```python
from build123d import *

# Parameters (mm, degrees)
SKETCH1_R               = 32.5
SKETCH1_R_2             = 30
BOSS_EXTRUDE1_DEPTH     = 140
CUT_REVOLVE1_ANGLE      = 67
CUT_REVOLVE2_ANGLE      = 67
CUT_EXTRUDE1_DEPTH      = 58
CUT_EXTRUDE1_DEPTH_BACK = 50
BOSS_EXTRUDE3_START     = -70
SKETCH4_R               = 1.55
BOSS_EXTRUDE3_DEPTH     = 4
SKETCH6_W               = 19.62
SKETCH6_H               = 2.5
BOSS_EXTRUDE4_DEPTH     = 6
SKETCH7_W               = 6
SKETCH7_H               = 9.773229536
BOSS_EXTRUDE6_DEPTH     = 3
SKETCH8_W               = 2.5
SKETCH8_H               = 1.33
BOSS_EXTRUDE7_DEPTH     = 6
SKETCH9_R               = 1.1
CUT_EXTRUDE2_DEPTH      = 7
RIB3_REACH              = 156.088
SKETCH11_WALL_W         = 347.41014935
SKETCH11_WALL_H         = 6


with BuildPart() as part:
    # Sketch1 → Boss-Extrude1 (new body)
    with BuildSketch(Plane(origin=(0, 0, 0), x_dir=(1, 0, 0), z_dir=(0, 1, 0))):
        with Locations(Location((0, 0, 0), (0, 0, 270))):
            Circle(SKETCH1_R)
        with Locations(Location((0, 0, 0), (0, 0, 270))):
            Circle(SKETCH1_R_2, mode=Mode.SUBTRACT)
    extrude(amount=BOSS_EXTRUDE1_DEPTH)

    # Sketch2 → Cut-Revolve1 (revolve, cut)
    with BuildSketch(Plane.XY):
        with BuildLine():
            Line((-42.5, 107.716148379), (42.5, 107.716148379))
            ThreePointArc((42.5, 107.716148379), (0, 150.216148379), (-42.5, 107.716148379))
        make_face()
    revolve(axis=Axis((-42.5, 107.716148379, 0), (1, 0, 0)), revolution_arc=CUT_REVOLVE1_ANGLE, mode=Mode.SUBTRACT)

    # Sketch3 → Cut-Revolve2 (revolve, cut)
    with BuildSketch(Plane.XY):
        with BuildLine():
            Line((-42.5, 70.076349177), (42.5, 70.076349177))
            ThreePointArc((42.5, 70.076349177), (0, 27.576349177), (-42.5, 70.076349177))
        make_face()
    revolve(axis=Axis((-42.5, 70.076349177, 0), (1, 0, 0)), revolution_arc=CUT_REVOLVE2_ANGLE, mode=Mode.SUBTRACT)

    # Sketch5 → Cut-Extrude1 (cut, two sides)
    with BuildSketch(Plane(origin=(0, 0, 0), x_dir=(0, 0, -1), z_dir=(1, 0, 0))) as cut_extrude1_sk:
        with BuildLine():
            Line((-38.488633311, 38.604979811), (-38.087882821, 37.828391715))
            ThreePointArc((-38.087882821, 37.828391715), (-30.720780367, 29.920302027), (-20.314824517, 27))
            Line((-20.314824517, 27), (-19.990167054, 27))
            Line((-19.990167054, 27), (0, 27))
            Line((0, 27), (0, 5))
            Line((0, 5), (-38.488633311, 5))
            Line((-38.488633311, 5), (-38.488633311, 38.604979811))
        make_face()
    extrude(amount=CUT_EXTRUDE1_DEPTH, mode=Mode.SUBTRACT)
    extrude(cut_extrude1_sk.sketch, amount=-CUT_EXTRUDE1_DEPTH_BACK, mode=Mode.SUBTRACT)

    # Sketch4 → Boss-Extrude3 (add)
    with BuildSketch(Plane(origin=(0, 140, 0), x_dir=(1, 0, 0), z_dir=(0, 1, 0)).offset(BOSS_EXTRUDE3_START)):
        with BuildLine():
            Line((-2.218998773, 40.206666667), (-20.604988608, 25.133333333))
            ThreePointArc((-20.604988608, 25.133333333), (0, 32.5), (20.604988608, 25.133333333))
            Line((20.604988608, 25.133333333), (2.218998773, 40.206666667))
            ThreePointArc((2.218998773, 40.206666667), (0, 41), (-2.218998773, 40.206666667))
        make_face()
        with Locations(Location((0, 37.5, 0), (0, 0, 270))):
            Circle(SKETCH4_R, mode=Mode.SUBTRACT)
        with BuildLine():
            ThreePointArc((-25.133333333, -20.604988608), (-32.5, 0), (-25.133333333, 20.604988608))
            Line((-25.133333333, 20.604988608), (-40.206666667, 2.218998773))
            ThreePointArc((-40.206666667, 2.218998773), (-41, 0), (-40.206666667, -2.218998773))
            Line((-40.206666667, -2.218998773), (-25.133333333, -20.604988608))
        make_face()
        with Locations(Location((-37.5, 0, 0), (0, 0, 270))):
            Circle(SKETCH4_R, mode=Mode.SUBTRACT)
        with BuildLine():
            Line((40.206666667, 2.218998773), (25.133333333, 20.604988608))
            ThreePointArc((25.133333333, 20.604988608), (32.5, 0), (25.133333333, -20.604988608))
            Line((25.133333333, -20.604988608), (40.206666667, -2.218998773))
            ThreePointArc((40.206666667, -2.218998773), (41, 0), (40.206666667, 2.218998773))
        make_face()
        with Locations(Location((37.5, 0, 0), (0, 0, 270))):
            Circle(SKETCH4_R, mode=Mode.SUBTRACT)
        with BuildLine():
            ThreePointArc((20.604988608, -25.133333333), (0, -32.5), (-20.604988608, -25.133333333))
            Line((-20.604988608, -25.133333333), (-2.218998773, -40.206666667))
            ThreePointArc((-2.218998773, -40.206666667), (0, -41), (2.218998773, -40.206666667))
            Line((2.218998773, -40.206666667), (20.604988608, -25.133333333))
        make_face()
        with Locations(Location((0, -37.5, 0), (0, 0, 270))):
            Circle(SKETCH4_R, mode=Mode.SUBTRACT)
    extrude(amount=-BOSS_EXTRUDE3_DEPTH)

    # Sketch6 → Boss-Extrude4 (add)
    with BuildSketch(Plane.XY):
        with Locations((39.81, 24.42)):
            Rectangle(SKETCH6_W, SKETCH6_H)
    extrude(amount=BOSS_EXTRUDE4_DEPTH)

    # Sketch7 → Boss-Extrude6 (add)
    with BuildSketch(Plane(origin=(49.62, 0, 0), x_dir=(0, 0, -1), z_dir=(1, 0, 0))):
        with Locations((-3, 18.283385232)):
            Rectangle(SKETCH7_W, SKETCH7_H)
    extrude(amount=-BOSS_EXTRUDE6_DEPTH)

    # Sketch8 → Boss-Extrude7 (add)
    with BuildSketch(Plane.XY):
        Polygon((49.62, 25.67), (32.5, 25.67), (32.5, 27), align=None)
        with Locations((31.25, 26.335)):
            Rectangle(SKETCH8_W, SKETCH8_H)
    extrude(amount=BOSS_EXTRUDE7_DEPTH)

    # Sketch9 → Cut-Extrude2 (cut)
    with BuildSketch(Plane(origin=(49.62, 0, 0), x_dir=(0, 0, -1), z_dir=(1, 0, 0))):
        with Locations((-3, 14.913761398)):
            Circle(SKETCH9_R)
    extrude(amount=-CUT_EXTRUDE2_DEPTH, mode=Mode.SUBTRACT)

    # Sketch11 wall → Rib3 (add, up to next)
    with BuildSketch(Plane(origin=(41.06, 42.202329556, 0), x_dir=(0.459795586238, -0.888024785057, 0), z_dir=(0.888024785057, 0.459795586238, 0)), mode=Mode.PRIVATE) as rib3_sk1:
        with Locations((0, -3)):
            Rectangle(SKETCH11_WALL_W, SKETCH11_WALL_H)
    rib3_tool1 = extrude(rib3_sk1.sketch, amount=-RIB3_REACH, mode=Mode.PRIVATE) - part.part
    add(rib3_tool1.solids().sort_by_distance((41.06, 42.202329556, 0))[0])


solid = part.part
```
Geometry check sheet. Reference: the model listing, model coordinates, mm. A direction names the side the tool comes from. Round coordinates to 2 decimals unless told otherwise and drop trailing zeros. Loops run counter-clockwise (first coordinate to the right, second up) from the corner with the lowest first, then second, coordinate; pieces in that order, holes last. Notation, with made-up numbers: (-12, 73) -> (1, 73) arc R18 cw to (1, 89) -> close; hole circle Ø5 at (46, 24). An arc over 180 degrees is marked (long way). Use a Markdown table: item, result.
(1) Set-up check for faces 4 (the flat face through (46.62, 18, 3)), 5 (the flat face through (0, 5, 31)), 6 (the cylindrical face through (21.97, 69.02, -23.95)), 7 (the cylindrical face through (41, 68, 0)), 8 (the cylindrical face through (35.987, 68.028, -0.336)): record each of +Z, -Z, +X, -X, +Y, -Y from which the full face is reachable in a straight line by a thin tool's end or side.
Calculated:
| item | result |
|---|---|
| face 4 | +Z, -Z, -X, -Y |
| face 5 | +Z, +X, -X |
| face 6 | none |
| face 7 | +X, +Y |
| face 8 | +Y |
(2) Go/stop test with flat-tipped pins: P1, Ø8, axis at x = -34, z = -7, coming from the -Y side; P2, Ø2.5, axis at x = 37.5, z = 0, coming from the -Y side; P3, Ø8, axis at x = -15, y = 78.5, coming from the +Z side; P4, Ø1.9, axis at y = 25, z = 2, coming from the -X side. Record where each tip stops, or that it passes through.
Calculated:
| item | result |
|---|---|
| P1 | y = 0 |
| P2 | y = 23.17 |
| P3 | z = 30.58 |
| P4 | x = 30 |
(3) Scan lines: probe 1 along X at (y, z) = (48.5, 17); probe 2 along X at (y, z) = (74.5, 26); probe 3 along Z at (x, y) = (-37, 68). Record each from-to range of solid material in increasing order.
Calculated:
| item | result |
|---|---|
| probe 1 | -27.7 to -24.72, 24.72 to 27.7 |
| probe 2 | -19.5 to -14.97, 14.97 to 19.5 |
| probe 3 | -6.13 to -1.47, 1.47 to 6.13 |
(4) Sectioned sample at A-A (x = 12.5). Enter the section's corners in (y, z), then the cut area to 3 significant figures.
Calculated:
| item | result |
|---|---|
| outline | (0, -30) -> (42.69, -30) arc R40.62 cw to (39.97, -27.27) -> (0, -27.27) -> close; (0, 27.27) -> (5, 27.27) -> (5, 30) -> (0, 30) -> close; (28.25, 27.27) -> (119.29, 27.27) -> (120.45, 30) -> (70, 30) -> (70, 31.78) -> (66, 31.78) -> (66, 30) -> (29.5, 30) arc R20 ccw to start; (57.34, -30) -> (66, -30) -> (66, -31.78) -> (70, -31.78) -> (70, -30) -> (140, -30) -> (140, -27.27) -> (58.5, -27.27) -> close; (135.1, 30) arc R40.62 cw to (137.82, 27.27) -> (140, 27.27) -> (140, 30) -> close |
| area | 622 mm² |
(5) Sectioned sample at C-C (x = -37.5). Enter the section's corners in (y, z).
Calculated:
| item | result |
|---|---|
| outline | (66, -5.52) -> (70, -5.52) -> (70, -1.55) -> (66, -1.55) -> close; (66, 1.55) -> (70, 1.55) -> (70, 5.52) -> (66, 5.52) -> close |
(6) Sectioned sample at D-D (z = -37.5). Enter the section's corners in (x, y), then the cut area to 3 significant figures.
Calculated:
| item | result |
|---|---|
| outline | (-5.52, 66) -> (-1.55, 66) -> (-1.55, 70) -> (-5.52, 70) -> close; (1.55, 66) -> (5.52, 66) -> (5.52, 70) -> (1.55, 70) -> close |
| area | 31.8 mm² |
(7) Mould release check, pull along Y, two halves, no side actions. Record for faces 1 (the flat face through (-28.4, 27, 11)), 2 (the cylindrical face through (-41, 68, 0)), 3 (the flat face through (-29, 0, 9)): released by +Y, released by -Y, zero draft, split by the parting line, or undercut.
Calculated:
| item | result |
|---|---|
| face 1 | undercut |
| face 2 | zero draft |
| face 3 | released by -Y |
(8) Sectioned sample at B-B (z = 15). Give the number of separate pieces and of enclosed holes in the cut face, then the cut area to 3 significant figures.
Calculated:
| item | result |
|---|---|
| separate pieces | 6 |
| enclosed holes | 0 |
| area | 552 mm² |
